Autodesk Inventor part; units mm, degrees
ref_plane "YZ Plane" through (0, 0, 0) normal (1, 0, 0) x (0, 1, 0)
ref_plane "XZ Plane" through (0, 0, 0) normal (0, 1, 0) x (-1, 0, 0)
ref_plane "XY Plane" through (0, 0, 0) normal (0, 0, 1) x (1, 0, 0)
sketch "Sketch1" plane through (0, 0, 0) normal (0, 0, 1) x (1, 0, 0)
  line L0 (76.2, 0) -> (0, 0)
  line L1 (0, 0) -> (0, 76.2)
  line L2 (0, 76.2) -> (25.4, 76.2)
  line L3 (25.4, 76.2) -> (76.2, 25.4)
  line L4 (76.2, 25.4) -> (76.2, 0)
  point P0 (12.7, 63.5)
  point P1 (12.7, 38.1)
  point P2 (12.7, 12.7)
  point P3 (38.1, 12.7)
  point P4 (63.5, 12.7)
  dimension "d0" = 76.2
  dimension "d1" = 76.2
  dimension "d2" = 25.4
  dimension "d3" = 25.4
  dimension "d4" = 12.7
  dimension "d5" = 12.7
  dimension "d6" = 25.4
  dimension "d7" = 25.4
  dimension "d8" = 25.4
  dimension "d9" = 25.4
extrude "Extrusion1" add sketch "Sketch1" against normal blind 4.7625
hole "Hole1" at (12.7, 63.5, 0) at (12.7, 38.1, 0) at (12.7, 12.7, 0) at (38.1, 12.7, 0) at (63.5, 12.7, 0) direction (0, 0, -1) diameter 6.35 depth 25.4 tip angle 118
properties part number "8020_gussetplate"
Work out the finished part from the listing and answer in its coordinate system (mm). Give positions to 0.01 mm unless a question says otherwise; leave off trailing zeros. Write each loop counter-clockwise with the first axis right and the second up, starting at its lowest first coordinate (ties: lowest second). Pieces come first, ordered by that corner, then holes. Notation, with made-up numbers: (-6.75, 8.25) -> (41.25, 8.25) arc R4 ccw to (41.25, 15.25) -> close; hole circle Ø7 at (46, -38.75). An arc over 180 degrees is marked (long way). Write item = value, one per line.
Q1. Section B-B on x = 38.1 is taken. Determine the outline of the cut face in (y, z) (1 decimal).
Computed values:
outline = (0, -4.8) -> (9.5, -4.8) -> (9.5, 0) -> (0, 0) -> close; (15.9, -4.8) -> (63.5, -4.8) -> (63.5, 0) -> (15.9, 0) -> close
Q2. Section A-A on y = 12.7 is taken. Determine the outline of the cut face in (x, z) (1 decimal).
Computed values:
outline = (0, -4.8) -> (9.5, -4.8) -> (9.5, 0) -> (0, 0) -> close; (15.9, -4.8) -> (34.9, -4.8) -> (34.9, 0) -> (15.9, 0) -> close; (41.3, -4.8) -> (60.3, -4.8) -> (60.3, 0) -> (41.3, 0) -> close; (66.7, -4.8) -> (76.2, -4.8) -> (76.2, 0) -> (66.7, 0) -> close
Q3. Section C-C on z = -1.9 is taken. Determine the outline of the cut face in (x, y) (3 decimals).
Computed values:
outline = (0, 0) -> (76.2, 0) -> (76.2, 25.4) -> (25.4, 76.2) -> (0, 76.2) -> close; hole circle Ø6.35 at (12.7, 12.7); hole circle Ø6.35 at (12.7, 38.1); hole circle Ø6.35 at (12.7, 63.5); hole circle Ø6.35 at (38.1, 12.7); hole circle Ø6.35 at (63.5, 12.7)
Q4. For a pull along Y with two mould halves and no side action, classify faces 1 (the cylindrical face through (12.56, 41.27, -2.41)), 2 (the cylindrical face through (35.423, 10.993, -2.415)), 3 (the flat face through (13, 76.2, -2)), 4 (the flat face through (0, 38, -2)) as pulls with the +Y half, pulls with the -Y half, needs draft (parallel to the pull), parting line crosses it, or undercut.
Computed values:
face_1 = undercut
face_2 = undercut
face_3 = pulls with the +Y half
face_4 = needs draft
Q5. Flat-ended cylindrical pins translate along their axes: pin 1 Ø1.5 at (x, z) = (51.5, -0.5) entering from +Y; pin 2 Ø12 at (x, y) = (56.5, 45) entering from +Z. Find the tip coordinate at first contact, or state that the pin passes through.
Computed values:
pin_1 = 50.85
pin_2 = 0
Q6. Consider line 1 along X through (y, z) = (12.7, -3.05) (3 decimals); line 2 along Y through (x, z) = (10, -1.95). Determine where each line is inside the solid, lowest interval first.
Computed values:
line_1 = 0 to 9.525, 15.875 to 34.925, 41.275 to 60.325, 66.675 to 76.2
line_2 = 0 to 11.03, 14.37 to 36.43, 39.77 to 61.83, 65.17 to 76.2
